For this review, use the dimensioned drawing (mm, ordinates from the lowest corner) and the shaded views. Give positions to 0.01 mm unless a question says otherwise; leave off trailing zeros. Order: outer loops, then holes, each group sorted by start corner. A loop starts at its lowest first (then second) coordinate and runs counter-clockwise, first axis right, second up. Notation, with made-up numbers: M -11.5,80 L 7.5,80 A24 ccw 7.5,117 Z; hole C -40,-19.75 d3. An arc over 180 degrees is marked long. Use CSV: the item, a comma, the result in double quotes. Start each with the question number.
(1) Clearance check with flat-ended pins moving along their axes: P1, Ø12, axis at x = 17.5, y = 6, coming from the -Z side; P2, Ø1.5, axis at x = 14.5, z = 5, coming from the +Y side; P3, Ø3, axis at x = 14.5, y = 14.5, coming from the +Z side; P4, Ø6, axis at y = 16, z = 21.5, coming from the -X side. State where each tip first meets the part, or that it passes through.
(2) Wall thickness on L1, parallel to Y at x = 12.5, z = 13; L2, parallel to X at y = 8.5, z = 13.5; L3, parallel to X at y = 9, z = 7.75: over which ranges is each line inside the solid? List them lowest first. Write a range as from..to.
(3) Consider section C-C (z = 6.75). Write out the cut boundary in (x, y).
(4) Draft analysis for pull direction Y (two halves, no side actions). For the marked faces 1, 2 and 3, state which applies: pulls with the +Y half, pulls with the -Y half, needs draft (parallel to the pull), parting line crosses it, or undercut.
(5) Consider section A-A (y = 12.5). Write out the cut boundary in (x, z), and give its area (3 significant figures).
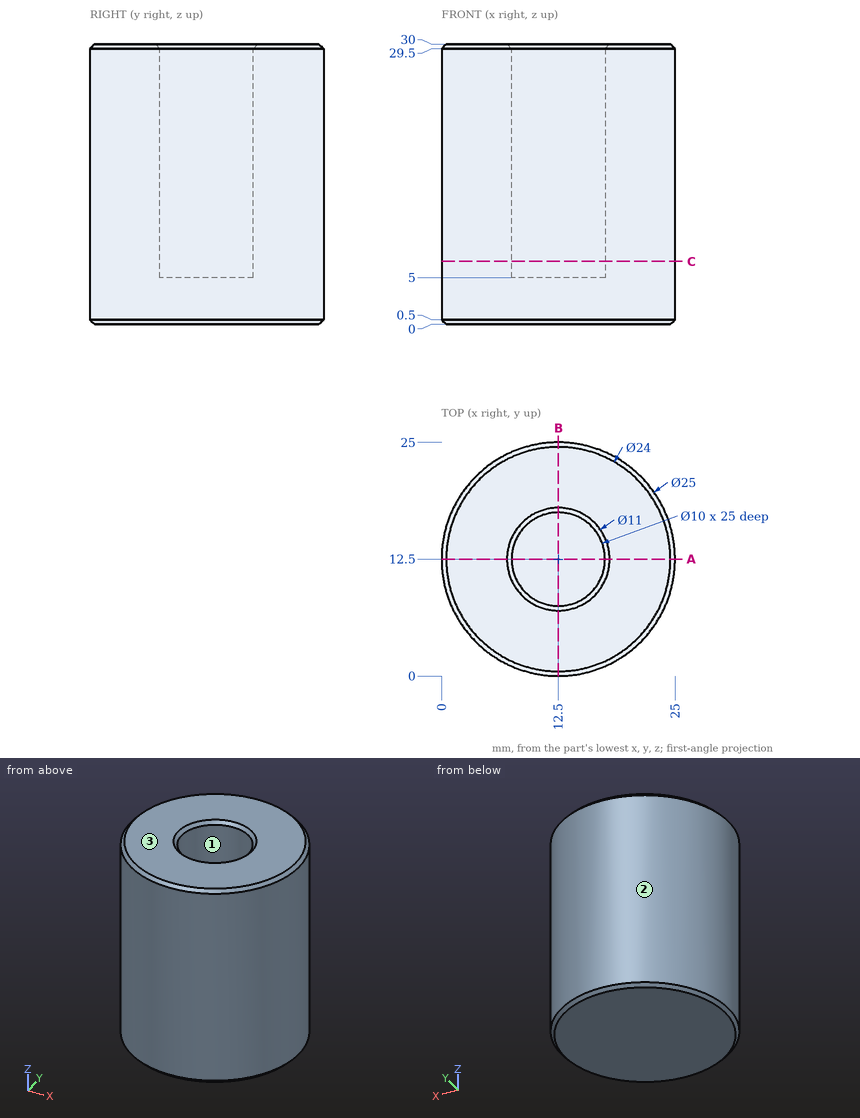
Check result:
1,P1,"stops at z = 0"
1,P2,"stops at y = 24.94"
1,P3,"stops at z = 5"
1,P4,"stops at x = 0.01"
2,L1,"y = 0..7.5, 17.5..25"
2,L2,"x = 0.66..9.5, 15.5..24.34"
2,L3,"x = 0.5..8.93, 16.07..24.5"
3,outline,"C 12.5,12.5 d25; hole C 12.5,12.5 d10"
4,face 1,"undercut"
4,face 2,"parting line crosses it"
4,face 3,"needs draft"
5,outline,"M 0,0.5 L 0.5,0 L 24.5,0 L 25,0.5 L 25,29.5 L 24.5,30 L 18,30 L 17.5,29.5 L 17.5,5 L 7.5,5 L 7.5,29.5 L 7,30 L 0.5,30 L 0,29.5 Z"
5,area,"499 mm^2"
